Autodesk Inventor part; units mm, degrees
ref_plane "YZ Plane" through (0, 0, 0) normal (1, 0, 0) x (0, 1, 0)
ref_plane "XZ Plane" through (0, 0, 0) normal (0, 1, 0) x (-1, 0, 0)
ref_plane "XY Plane" through (0, 0, 0) normal (0, 0, 1) x (1, 0, 0)
sketch "Sketch2" plane through (0, 0, 0) normal (0, 0, 1) x (1, 0, 0)
  line L0 (-70, 20) -> (-70, -20)
  line L1 (-70, -20) -> (-50, -20)
  line L2 (-50, -20) -> (-50, -25)
  line L3 (-50, -25) -> (-10, -25)
  line L4 (-10, -25) -> (-10, -20)
  line L5 (-10, -20) -> (10, -20)
  line L6 (10, -20) -> (10, -25)
  line L7 (10, -25) -> (50, -25)
  line L8 (50, -25) -> (50, -20)
  line L9 (50, -20) -> (70, -20)
  line L10 (70, -20) -> (70, 20)
  line L11 (70, 20) -> (50, 20)
  line L12 (50, 20) -> (50, 25)
  line L13 (50, 25) -> (10, 25)
  line L14 (10, 25) -> (10, 20)
  line L15 (10, 20) -> (-10, 20)
  line L16 (-10, 20) -> (-10, 25)
  line L17 (-10, 25) -> (-50, 25)
  line L18 (-50, 25) -> (-50, 20)
  line L19 (-50, 20) -> (-70, 20)
  point P0 (0, 0)
  point P1 (0, 20)
  point P2 (0, -20)
  point P3 (-70, 0)
  point P4 (70, 0)
  dimension "d11" = 5
  dimension "d12" = 40
  dimension "d13" = 20
  dimension "d14" = 40
  dimension "d15" = 140
  dimension "d16" = 40
  dimension "d17" = 5
  dimension "d18" = 70
extrude "Extrusion1" add sketch "Sketch2" along normal blind 5
sketch "Sketch3" plane through (0, 0, 5) normal (0, 0, 1) x (1, 0, 0)
  line L0 (10, 20) -> (-10, 20)
  line L1 (-10, -20) -> (10, -20)
  line L2 (1.6, 20) -> (-1.6, 20)
  line L3 (-1.6, 20) -> (-1.6, 16.9)
  line L4 (-1.6, 16.9) -> (-2.75, 16.9)
  line L5 (-2.75, 16.9) -> (-2.75, 14.5)
  line L6 (-2.75, 14.5) -> (2.75, 14.5)
  line L7 (2.75, 14.5) -> (2.75, 16.9)
  line L8 (2.75, 16.9) -> (1.6, 16.9)
  line L9 (1.6, 20) -> (1.6, 16.9)
  line L10 (-1.6, -20) -> (1.6, -20)
  line L11 (1.6, -20) -> (1.6, -16.9)
  line L12 (1.6, -16.9) -> (2.75, -16.9)
  line L13 (2.75, -16.9) -> (2.75, -14.5)
  line L14 (2.75, -14.5) -> (-2.75, -14.5)
  line L15 (-2.75, -14.5) -> (-2.75, -16.9)
  line L16 (-2.75, -16.9) -> (-1.6, -16.9)
  line L17 (-1.6, -16.9) -> (-1.6, -20)
  point P0 (0, 0)
  point P1 (0, 20)
  point P2 (0, 14.5)
  point P3 (0, -20)
  point P4 (0, -14.5)
  point P5 (0, 20)
  dimension "d21" = 3.2
  dimension "d22" = 2.4
  dimension "d23" = 2.4
  dimension "d24" = 3.2
  dimension "d25" = 5.5
  dimension "d26" = 5.5
  dimension "d27" = 5.5
  dimension "d28" = 5.5
extrude "Extrusion2" cut sketch "Sketch3" against normal blind 5
properties part number "Interrupter_Side" material "Polycarbonate, Clear"
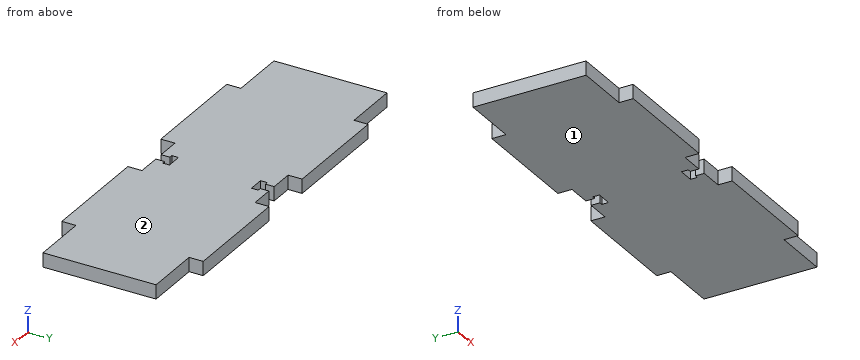
Model file for the job. Use its own axes, mm. Face numbers are marked on the shaded views. Give positions to 0.01 mm unless a question says otherwise; leave off trailing zeros. Write each loop counter-clockwise with the first axis right and the second up, starting at its lowest first coordinate (ties: lowest second). Pieces come first, ordered by that corner, then holes. Notation, with made-up numbers: M -39,-5 L 15,-5 A26 ccw 15,24 Z; hole C 79.25,15.25 d6. An arc over 180 degrees is marked long. Use a Markdown table: item, result.
1) Pin check, flat tips, straight feed: pin 1 (5 mm diameter, centred on x = 7, y = 3.5, fed in from -Z); pin 2 (1.5 mm diameter, centred on x = -5, z = 3, fed in from -Y); pin 3 (1.5 mm diameter, centred on x = -7.5, z = 2.5, fed in from +Y); pin 4 (1.5 mm diameter, centred on y = -21.5, z = 1.5, fed in from -X). Stop position of each tip, or through.
Responses:
| item | result |
|---|---|
| pin 1 | stops at z = 0 |
| pin 2 | stops at y = -20 |
| pin 3 | stops at y = 20 |
| pin 4 | stops at x = -50 |
2) Pull direction Z, two halves, no side cores. Call the marked faces 1 and 2: +Z half, -Z half, draft (parallel to the pull), parting line (faces both ways), or undercut.
Responses:
| item | result |
|---|---|
| face 1 | -Z half |
| face 2 | +Z half |
3) Drill centre lines: line 1 (X direction, y = 19.5, z = 0.85); line 2 (X direction, y = 16, z = 1.9); line 3 (Y direction, x = 5.5, z = 4.6). Where is each one in solid material? Low to high. Write a range as from..to.
Responses:
| item | result |
|---|---|
| line 1 | x = -70..-1.6, 1.6..70 |
| line 2 | x = -70..-2.75, 2.75..70 |
| line 3 | y = -20..20 |
4) Cut at B-B (x = 57.5). List the corners of the cut face in (y, z), and give its area (3 significant figures).
Responses:
| item | result |
|---|---|
| outline | M -20,0 L 20,0 L 20,5 L -20,5 Z |
| area | 200 mm2 |
5) Cut at A-A (y = 18.5). List the corners of the cut face in (x, z).
Responses:
| item | result |
|---|---|
| outline | M -70,0 L -1.6,0 L -1.6,5 L -70,5 Z; M 1.6,0 L 70,0 L 70,5 L 1.6,5 Z |
